from build123d import *


with BuildPart() as part:
    # Эскиз1 → Повернуть1 (revolve)
    with BuildSketch(Plane.XY):
        with BuildLine():
            Line((0, 7), (0, 13))
            ThreePointArc((0, 13), (-0.292893219, 13.707106781), (-1, 14))
            Line((-1, 14), (-7, 14))
            ThreePointArc((-7, 14), (-7.707106781, 13.707106781), (-8, 13))
            Line((-8, 13), (-8, 7))
            ThreePointArc((-8, 7), (-7.707106781, 6.292893219), (-7, 6))
            Line((-7, 6), (-1, 6))
            ThreePointArc((-1, 6), (-0.292893219, 6.292893219), (0, 7))
        make_face()
    revolve(axis=Axis((0, 0, 0), (-1, 0, 0)))


solid = part.part
Build history of the part. All positions in model axes, mm. Round coordinates to 2 decimals unless told otherwise and drop trailing zeros. Order: outer loops, then holes, each group sorted by start corner. A loop starts at its lowest first (then second) coordinate and runs counter-clockwise, first axis right, second up. Notation, with made-up numbers: M -27.75,24 L 6.25,24 A13 ccw 6.25,49 Z; hole C 88.25,-34.75 d5. An arc over 180 degrees is marked long. Use CSV: the item, a comma, the result in double quotes. Start each with the question number.
(1) Flat gauge pins, fed straight in: P1, Ø1, axis at x = -5, y = -10.5, coming from the -Z side; P2, Ø4, axis at x = -6, z = -7, coming from the -Y side; P3, Ø1.5, axis at y = 8, z = -1, coming from the +X side; P4, Ø1, axis at x = -7, y = 10.5, coming from the +Z side. Where does each tip first touch, or does it go through?
(2) Cut at A-A on y = 0. List the corners of the cut face in (x, z), then the cut area to 3 significant figures.
(3) Mould opens along Y. For faces 1 (the face through (-4, -6, 0)), 2 (the face through (0, -6, 6)), 3 (the face through (-4.042, 12.932, 5.362)) say: +Y half, -Y half, draft (parallel to the pull), parting line (faces both ways), or undercut.
(4) Cut at C-C on x = -5.5. List the corners of the cut face in (y, z), then the cut area to 3 significant figures.
(5) Drill centre lines: probe 1 along Z at (x, y) = (-3.9, 0); probe 2 along X at (y, z) = (12.5, 3.75). Where is each one in solid material? Low to high.
Findings:
1,P1,"stops at z = -9.8"
1,P2,"stops at y = -13.08"
1,P3,"stops at x = 0"
1,P4,"stops at z = 9.8"
2,outline,"M -8,-13 A1 ccw -7,-14 L -1,-14 A1 ccw 0,-13 L 0,-7 A1 ccw -1,-6 L -7,-6 A1 ccw -8,-7 Z; M -8,7 A1 ccw -7,6 L -1,6 A1 ccw 0,7 L 0,13 A1 ccw -1,14 L -7,14 A1 ccw -8,13 Z"
2,area,"126 mm^2"
3,face 1,"undercut"
3,face 2,"draft"
3,face 3,"parting line"
4,outline,"C 0,0 d28; hole C 0,0 d12"
4,area,"503 mm^2"
5,probe 1,"z = -14 to -6, 6 to 14"
5,probe 2,"x = -8 to 0"
